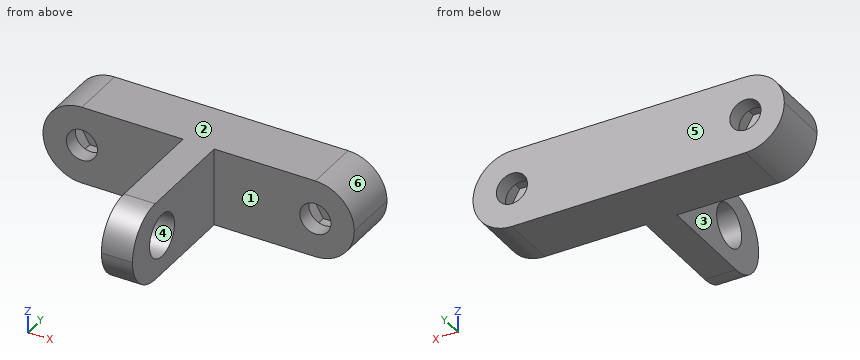
```python
from build123d import *

# Parameters (mm, degrees)
F0_W     = 40
F0_H     = 10
F0_R     = 2
F1_DEPTH = 2
F2_W     = 40
F2_H     = 10
F3_DEPTH = 3.2
F4_START = 5.2
F4_DEPTH = 2
F5_W     = 4
F5_H     = 10
F6_DEPTH = 18
F7_R     = 2.75
F8_DEPTH = 25
F9_R     = 4.99999


# Not quite as in the source:
# - a fillet or chamfer is up to 0.001 mm smaller than in the source, because OpenCascade refuses the exact size


with BuildPart() as f1:
    # F0 (on Front) → F1 (new body)
    with BuildSketch(Plane.XZ):
        Rectangle(F0_W, F0_H)
        with Locations((-15, 0)):
            Circle(F0_R, mode=Mode.SUBTRACT)
        with Locations((15, 0)):
            Circle(F0_R, mode=Mode.SUBTRACT)
    extrude(amount=F1_DEPTH)

    # F2 (on face) → F3 (join)
    with BuildSketch(Plane.XZ.offset(2)):
        Rectangle(F2_W, F2_H)
        Polygon((-10.9585481157, 0), (-12.9792740578, -3.5), (-17.0207259422, -3.5), (-19.0414518843, 0), (-17.0207259422, 3.5), (-12.9792740578, 3.5), align=None, mode=Mode.SUBTRACT)
        Polygon((19.0414518843, 0), (17.0207259422, -3.5), (12.9792740578, -3.5), (10.9585481157, 0), (12.9792740578, 3.5), (17.0207259422, 3.5), align=None, mode=Mode.SUBTRACT)
    extrude(amount=F3_DEPTH)

    # F0 (on Front) → F4 (join)
    with BuildSketch(Plane.XZ.offset(F4_START)):
        Rectangle(F0_W, F0_H)
        with Locations((-15, 0)):
            Circle(F0_R, mode=Mode.SUBTRACT)
        with Locations((15, 0)):
            Circle(F0_R, mode=Mode.SUBTRACT)
    extrude(amount=F4_DEPTH)

    # F5 (on face) → F6 (join)
    with BuildSketch(Plane.XZ.offset(7.2)):
        Rectangle(F5_W, F5_H)
    extrude(amount=F6_DEPTH)

    # F7 (on face) → F8 (cut)
    with BuildSketch(Plane.YZ.offset(2)):
        with Locations((-18.7, 0)):
            Circle(F7_R)
    extrude(amount=-F8_DEPTH, mode=Mode.SUBTRACT)

    # F9 (radius 5 in the source; OpenCascade refuses exactly that, so slightly less here)
    f9_edges = [f1.edges().sort_by_distance(p)[0] for p in [
        (0, -25.2, 5),
        (0, -25.2, -5),
        (20, -3.6, 5),
        (20, -3.6, -5),
        (-20, -3.6, 5),
        (-20, -3.6, -5),
    ]]
    fillet(f9_edges, radius=F9_R)


solid = f1.part
```
Model file for the job. Use its own axes, mm. Face numbers are marked on the shaded views. A direction names the side the tool comes from. Coordinates: 2 decimals unless noted, no trailing zeros. Write each loop counter-clockwise with the first axis right and the second up, starting at its lowest first coordinate (ties: lowest second). Pieces come first, ordered by that corner, then holes. Notation, with made-up numbers: (30, 56.25) - (34, 56.25) arc R32 cw to (34, 95.25) - close; hole circle Ø11 at (16, 24.25). An arc over 180 degrees is marked (long way). Use a Markdown table: item, result. Add a question column.
Item 1: Drill centre lines: line 1 along Y through (x, z) = (-17, -2.25); line 2 along Z through (x, y) = (15, -1.5); line 3 along Y through (x, z) = (7, -1). Where is each one in solid material? Low to high.
Item 2: 3-axis set-ups, long thin cutter, end or side, ignore diameter. For the marked faces 1, 2 and 3: which of +Z, -Z, +X, -X, +Y, -Y reach the whole face in a straight line?
Item 3: Band-saw the part on D-D, the plane z = 4.5. Write the cut outline in (x, y).
Item 4: Two-plate mould, pull along Y, no slides. Class the marked faces 4, 5 and 6: pulls with the +Y half, pulls with the -Y half, needs draft (parallel to the pull), parting line crosses it, or undercut.
Item 5: Band-saw the part on A-A, the plane y = -18.7. Write the cut outline in (x, z).
Item 6: Band-saw the part on C-C, the plane x = -16.5. Write the cut outline in (y, z).
Item 7: Drop flat-ended pins along their axis: pin 1 (12 mm diameter, centred on x = 13.5, y = -15, fed in from +Z); pin 2 (3 mm diameter, centred on y = -19.5, z = -1.5, fed in from +X); pin 3 (5.5 mm diameter, centred on x = 16, z = -1.5, fed in from -Y); pin 4 (6 mm diameter, centred on y = -12, z = -2, fed in from -X). Give the stop position or say it passes through.
A:
| question | item | result |
|---|---|---|
| 1 | line 1 | y = -7.2 to -5.2, -2 to 0 |
| 1 | line 2 | z = -5 to -2, 2 to 5 |
| 1 | line 3 | y = -7.2 to 0 |
| 2 | face 1 | +Z, -Z, +X, -Y |
| 2 | face 2 | +Z, +X, -X, +Y, -Y |
| 2 | face 3 | +Z, -Z, -X, -Y |
| 3 | outline | (-17.18, -7.2) - (-2, -7.2) - (-2, -22.38) - (2, -22.38) - (2, -7.2) - (17.18, -7.2) - (17.18, 0) - (-17.18, 0) - close |
| 4 | face 4 | undercut |
| 4 | face 5 | pulls with the +Y half |
| 4 | face 6 | needs draft |
| 5 | outline | (-2, -5) - (2, -5) - (2, -2.75) - (-2, -2.75) - close; (-2, 2.75) - (2, 2.75) - (2, 5) - (-2, 5) - close |
| 6 | outline | (-7.2, -4.77) - (0, -4.77) - (0, -1.32) - (-2, -1.32) - (-2, -3.5) - (-5.2, -3.5) - (-5.2, -1.32) - (-7.2, -1.32) - close; (-7.2, 1.32) - (-5.2, 1.32) - (-5.2, 3.5) - (-2, 3.5) - (-2, 1.32) - (0, 1.32) - (0, 4.77) - (-7.2, 4.77) - close |
| 7 | pin 1 | passes through |
| 7 | pin 2 | stops at x = 2 |
| 7 | pin 3 | stops at y = -7.2 |
| 7 | pin 4 | stops at x = -2 |
